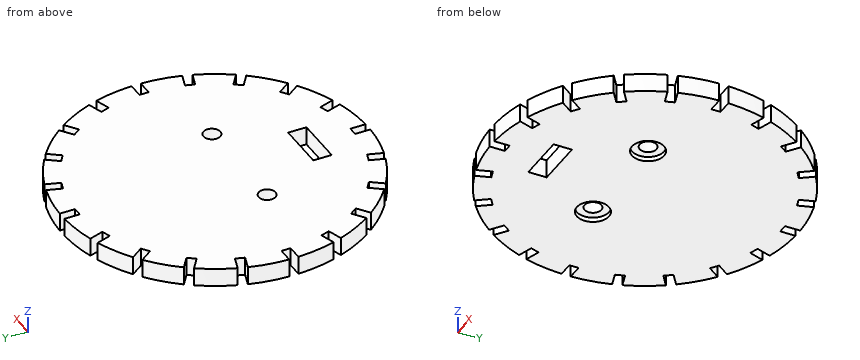
from build123d import *

# Parameters (mm, degrees)
SKETCH2_W           = 16
SKETCH2_H           = 6
SKETCH2_R           = 2.75
BOSS_EXTRUDE1_DEPTH = 6
SKETCH3_R           = 5.25
CUT_EXTRUDE1_DEPTH  = 1.5


with BuildPart() as part:
    # Sketch2 → Boss-Extrude1 (new body)
    with BuildSketch(Plane.XY):
        with BuildLine():
            ThreePointArc((-14.014958559, -48.70381072), (-7.820513245, -50.092784824), (-1.5, -50.685671098))
            Line((-1.5, -50.685671098), (-1.5, -45.708176163))
            Line((-1.5, -45.708176163), (1.5, -45.708176163))
            Line((1.5, -45.708176163), (1.5, -50.685671098))
            ThreePointArc((1.5, -50.685671098), (7.821643905, -50.09260576), (14.017156267, -48.703168924))
            Line((14.017156267, -48.703168924), (12.476730902, -43.962227135))
            Line((12.476730902, -43.962227135), (15.32990045, -43.035176152))
            Line((15.32990045, -43.035176152), (16.870328795, -47.776127109))
            ThreePointArc((16.870328795, -47.776127109), (22.700337229, -45.258088505), (28.164148211, -42.021379325))
            Line((28.164148211, -42.021379325), (25.229863981, -37.982683562))
            Line((25.229863981, -37.982683562), (27.656914964, -36.219327805))
            Line((27.656914964, -36.219327805), (30.591129228, -40.257927268))
            ThreePointArc((30.591129228, -40.257927268), (35.358240772, -36.060613271), (39.55477218, -31.292812793))
            Line((39.55477218, -31.292812793), (35.511033717, -28.354864828))
            Line((35.511033717, -28.354864828), (37.274389474, -25.927813845))
            Line((37.274389474, -25.927813845), (41.317825829, -28.865542317))
            ThreePointArc((41.317825829, -28.865542317), (44.554494815, -23.399517942), (47.071992795, -17.567224011))
            Line((47.071992795, -17.567224011), (42.313847582, -16.021208913))
            Line((42.313847582, -16.021208913), (43.240898565, -13.168039364))
            Line((43.240898565, -13.168039364), (47.998350807, -14.713829302))
            ThreePointArc((47.998350807, -14.713829302), (49.386863483, -8.514437454), (49.978066205, -2.189019992))
            Line((49.978066205, -2.189019992), (44.972398757, -2.189019992))
            Line((44.972398757, -2.189019992), (44.972398757, 0.810980008))
            Line((44.972398757, 0.810980008), (49.976916317, 0.810980008))
            ThreePointArc((49.976916317, 0.810980008), (49.380832331, 7.136146516), (47.987483994, 13.334664716))
            Line((47.987483994, 13.334664716), (43.22644973, 11.787710909))
            Line((43.22644973, 11.787710909), (42.299398746, 14.640880458))
            Line((42.299398746, 14.640880458), (47.058915168, 16.187341088))
            ThreePointArc((47.058915168, 16.187341088), (44.536626084, 22.0182168), (41.295318935, 27.482188044))
            Line((41.295318935, 27.482188044), (37.246906156, 24.540843989))
            Line((37.246906156, 24.540843989), (35.483550399, 26.967894972))
            Line((35.483550399, 26.967894972), (39.530326401, 29.908049839))
            ThreePointArc((39.530326401, 29.908049839), (35.329326435, 34.673156396), (30.558045552, 38.86714256))
            Line((30.558045552, 38.86714256), (27.619087422, 34.822013725))
            Line((27.619087422, 34.822013725), (25.192036439, 36.585369482))
            Line((25.192036439, 36.585369482), (28.129589934, 40.628565002))
            ThreePointArc((28.129589934, 40.628565002), (22.66202489, 43.861237429), (16.828745179, 46.374658668))
            Line((16.828745179, 46.374658668), (15.285431508, 41.62482759))
            Line((15.285431508, 41.62482759), (12.432261959, 42.551878573))
            Line((12.432261959, 42.551878573), (13.974753738, 47.299180128))
            ThreePointArc((13.974753738, 47.299180128), (7.776727495, 48.683346485), (1.453242586, 49.270700235))
            Line((1.453242586, 49.270700235), (1.453242586, 44.283378765))
            Line((1.453242586, 44.283378765), (-1.546757414, 44.283378765))
            Line((-1.546757414, 44.283378765), (-1.546757414, 49.2608737))
            ThreePointArc((-1.546757414, 49.2608737), (-7.866904098, 48.661958763), (-14.060191394, 47.266915506))
            Line((-14.060191394, 47.266915506), (-12.523488315, 42.537429737))
            Line((-12.523488315, 42.537429737), (-15.376657864, 41.610378754))
            Line((-15.376657864, 41.610378754), (-16.914659767, 46.343861891))
            ThreePointArc((-16.914659767, 46.343861891), (-22.740383136, 43.821308169), (-28.199510335, 40.580897657))
            Line((-28.199510335, 40.580897657), (-25.276621395, 36.557886164))
            Line((-25.276621395, 36.557886164), (-27.703672378, 34.794530407))
            Line((-27.703672378, 34.794530407), (-30.624981542, 38.815367524))
            ThreePointArc((-30.624981542, 38.815367524), (-35.385501758, 34.616974444), (-39.575762572, 29.849294558))
            Line((-39.575762572, 29.849294558), (-35.557791131, 26.93006743))
            Line((-35.557791131, 26.93006743), (-37.321146887, 24.503016447))
            Line((-37.321146887, 24.503016447), (-41.33714976, 27.420813327))
            ThreePointArc((-41.33714976, 27.420813327), (-44.567381262, 21.957845266), (-47.079571363, 16.129696634))
            Line((-47.079571363, 16.129696634), (-42.360604995, 14.596411515))
            Line((-42.360604995, 14.596411515), (-43.287655979, 11.743241967))
            Line((-43.287655979, 11.743241967), (-48.004645978, 13.275884924))
            ThreePointArc((-48.004645978, 13.275884924), (-49.389276358, 7.082804571), (-49.978315717, 0.764222594))
            Line((-49.978315717, 0.764222594), (-45.01915617, 0.764222594))
            Line((-45.01915617, 0.764222594), (-45.01915617, -2.235777406))
            Line((-45.01915617, -2.235777406), (-49.976658896, -2.235777406))
            ThreePointArc((-49.976658896, -2.235777406), (-49.380673152, -8.553500826), (-47.989286669, -14.744855434))
            Line((-47.989286669, -14.744855434), (-43.273207143, -13.212508307))
            Line((-43.273207143, -13.212508307), (-42.34615616, -16.065677856))
            Line((-42.34615616, -16.065677856), (-47.06108419, -17.597650839))
            ThreePointArc((-47.06108419, -17.597650839), (-44.542778803, -23.422507686), (-41.306963736, -28.881474636))
            Line((-41.306963736, -28.881474636), (-37.293663569, -25.965641387))
            Line((-37.293663569, -25.965641387), (-35.530307812, -28.39269237))
            Line((-35.530307812, -28.39269237), (-39.542974081, -31.308065065))
            ThreePointArc((-39.542974081, -31.308065065), (-35.348264075, -36.07058879), (-30.584062086, -40.263392586))
            Line((-30.584062086, -40.263392586), (-27.665844836, -36.246811123))
            Line((-27.665844836, -36.246811123), (-25.238793853, -38.01016688))
            Line((-25.238793853, -38.01016688), (-28.156765996, -42.026410983))
            ThreePointArc((-28.156765996, -42.026410983), (-22.695337069, -45.260635975), (-16.868173537, -47.776899552))
            Line((-16.868173537, -47.776899552), (-15.332188921, -43.049624988))
            Line((-15.332188921, -43.049624988), (-12.479019372, -43.976675971))
            Line((-12.479019372, -43.976675971), (-14.014958559, -48.70381072))
        make_face()
        with Locations((0, -31.708176163)):
            Rectangle(SKETCH2_W, SKETCH2_H, mode=Mode.SUBTRACT)
        with Locations((-17.5, -8.708176163)):
            Circle(SKETCH2_R, mode=Mode.SUBTRACT)
        with Locations((17.5, -8.708176163)):
            Circle(SKETCH2_R, mode=Mode.SUBTRACT)
    extrude(amount=BOSS_EXTRUDE1_DEPTH)

    # Sketch3 → Cut-Extrude1 (cut)
    with BuildSketch(Plane(origin=(0, 0, 0), x_dir=(-1, 0, 0), z_dir=(0, 0, -1))):
        with Locations((-17.5, -8.708176163)):
            Circle(SKETCH3_R)
        with Locations((17.5, -8.708176163)):
            Circle(SKETCH3_R)
    extrude(amount=-CUT_EXTRUDE1_DEPTH, mode=Mode.SUBTRACT)


solid = part.part
Geometry: final body of the model. Coordinates: model frame, mm. Round coordinates to 2 decimals unless told otherwise and drop trailing zeros. Loops run counter-clockwise (first coordinate to the right, second up) from the corner with the lowest first, then second, coordinate; pieces in that order, holes last. Notation, with made-up numbers: M 30,51 L 66,51 A6 ccw 66,61 Z; hole C 11.25,-9 d3. An arc over 180 degrees is marked long. One line per question, with ' | ' between items.
(1) Contact query for flat-ended pins moving along their axis: P1, Ø5, axis at x = -17.5, y = -8.71, coming from the -Z side; P2, Ø8, axis at x = -10, y = 26, coming from the -Z side; P3, Ø1.5, axis at y = -35.5, z = 3.5, coming from the -X side; P4, Ø1.5, axis at x = 0, z = 2.5, coming from the -Y side. Output: stop coordinate, or through.
Check result:
P1: passes through | P2: stops at z = 0 | P3: stops at x = -36.62 | P4: stops at y = -45.71
(2) Material intervals for line 1 along X through (y, z) = (-46, 1.4); line 2 along Y through (x, z) = (28, 1.5); line 3 along Y through (x, z) = (38, 1.65) (3 decimals), sorted ascending. Write a range as from..to.
Check result:
line 1: x = -21.18..-16.29, -13.14..-1.5, 1.5..13.14, 16.29..21.18 | line 2: y = -42.13..-41.8, -36.69..35.35, 40.45..40.72 | line 3: y = -33.204..-30.163, -26.455..25.088, 28.796..31.788
(3) Cut plane A-A on z = 3.55. Give the number of separate pieces and of enclosed holes in the cut face, plus the area to 3 significant figures.
Check result:
separate pieces: 1 | enclosed holes: 3 | area: 7,410 mm2
(4) Cut plane B-B on y = -22.5. Return the cut outline in (x, z), plus the area to 3 significant figures.
Check result:
outline: M -45,0 L 45,0 L 45,6 L -45,6 Z | area: 540 mm2
